Could you check a few things on this model? Use its own coordinates, in mm. A direction names the side the tool comes from. Give positions to 0.01 mm unless a question says otherwise; leave off trailing zeros. Order: outer loops, then holes, each group sorted by start corner. A loop starts at its lowest first (then second) coordinate and runs counter-clockwise, first axis right, second up. Notation, with made-up numbers: (69.25, 26) -> (95.25, 26) arc R22 ccw to (95.25, 64) -> close; hole circle Ø11 at (78, -27). An arc over 180 degrees is marked (long way). One line per item, written item: value.
```python
from build123d import *

# Parameters (mm, degrees)
SKETCH_1_R               = 18.75
EXTRUDE_1_DEPTH          = 60
SKETCH_2_R               = 6
EXTRUDE_2_DEPTH          = 5
SKETCH_3_R               = 3
EXTRUDE_3_DEPTH          = 15.5
SKETCH_4_W               = 7.331861777
SKETCH_4_H               = 1.908292791
CUT_EXTRUDE_1_DEPTH      = 14.5
PATTERN_CIRCULAR_1_COUNT = 6


with BuildPart() as part:
    # 草图1 → 凸台-拉伸1 (new body)
    with BuildSketch(Plane.XY):
        Circle(SKETCH_1_R)
    extrude(amount=EXTRUDE_1_DEPTH)

    # 草图2 → 凸台-拉伸2 (add)
    with BuildSketch(Plane.XY.offset(60)):
        with Locations((0, 7)):
            Circle(SKETCH_2_R)
    extrude(amount=EXTRUDE_2_DEPTH)

    # 草图3 → 凸台-拉伸3 (add)
    with BuildSketch(Plane.XY.offset(65)):
        with Locations((0, 7)):
            Circle(SKETCH_3_R)
    extrude(amount=EXTRUDE_3_DEPTH)

    # 草图4 → 切除-拉伸1 (cut)
    with BuildSketch(Plane.XY.offset(80.5)):
        with Locations((-0.04202298, 10.454146396)):
            Rectangle(SKETCH_4_W, SKETCH_4_H)
    extrude(amount=-CUT_EXTRUDE_1_DEPTH, mode=Mode.SUBTRACT)

    # 草图6 → M3 螺纹孔1 (revolve, cut)
    with BuildSketch(Plane(origin=(0, 15.5, 60), x_dir=(0, -1, 0), z_dir=(1, 0, 0))):
        Polygon((0, 0), (0, 8.251075774), (1.25, 7.5), (1.25, 0), align=None)
    hole_wizard_m3_1 = revolve(axis=Axis((0, 15.5, 66.35), (0, 0, -1)), mode=Mode.SUBTRACT)

    # 阵列(圆周)1: M3 螺纹孔1 ×6 about axis
    pattern_circular_1_axis = Axis((0, 0, 0), (0, 0, 1))
    for i in range(1, PATTERN_CIRCULAR_1_COUNT):
        add(hole_wizard_m3_1.rotate(pattern_circular_1_axis, i * 360 / PATTERN_CIRCULAR_1_COUNT), mode=Mode.SUBTRACT)


solid = part.part
```
1) For P1, Ø1.5, axis at x = 0, y = 15.5, coming from the +Z side; P2, Ø8, axis at x = -7, z = 45, coming from the +Y side; P3, Ø2.5, axis at x = 0, z = 71.5, coming from the +Y side, each with a flat end and sliding along its axis, tell me the tip position at first contact or that it passes through.
Answer below:
P1: stops at z = 52.2
P2: stops at y = 18.51
P3: stops at y = 9.5
2) Suppose I cut it at D-D, the plane y = 0. Write out the boundary of the cut face in (x, z), then the cut area to 3 significant figures.
Answer below:
outline: (-18.75, 0) -> (18.75, 0) -> (18.75, 60) -> (-18.75, 60) -> close
area: 2,250 mm2
3) For faces 1 (the flat face through (0, 9.5, 73)), 2 (the flat face through (0, 0, 0)), 3 (the cylindrical face through (12.184, -7.587, 56.302)), which set-ups out of +Z, -Z, +X, -X, +Y, -Y let a thin tool reach every point of the face, with its end or its side?
Answer below:
face 1: +Z, +X, -X, +Y
face 2: -Z, +X, -X, +Y, -Y
face 3: +Z
4) Suppose I cut it at C-C, the plane x = 5. Write out the boundary of the cut face in (y, z).
Answer below:
outline: (-18.07, 0) -> (18.07, 0) -> (18.07, 60) -> (10.32, 60) -> (10.32, 65) -> (3.68, 65) -> (3.68, 60) -> (-18.07, 60) -> close
5) If I drill on line 1 along Y through (x, z) = (-14, 57); line 2 along X through (y, z) = (7.75, 56.5); line 3 along X through (y, z) = (-7, 57), over which ranges is the centre line in solid material (lowest first)?
Answer below:
line 1: y = -12.47 to -8.86, -6.64 to 6.64, 8.86 to 12.47
line 2: x = -17.07 to -14.67, -12.17 to 12.17, 14.67 to 17.07
line 3: x = -17.39 to -14.42, -12.42 to 12.42, 14.42 to 17.39
6) Suppose I cut it at B-B, the plane z = 64. Write out the boundary of the cut face in (x, y), then the cut area to 3 significant figures.
Answer below:
outline: circle Ø12 at (0, 7)
area: 113 mm2
7) We'd pull the mould along X, two halves only. Please class faces 4 (the cylindrical face through (-14.27, -6.83, 56.3)), 5 (the flat face through (1, 10, 65)), 6 (the cylindrical face through (-0.78, 12.95, 62.46)): +X half, -X half, draft (parallel to the pull), parting line (faces both ways), or undercut.
Answer below:
face 4: undercut
face 5: draft
face 6: parting line
8) Suppose I cut it at A-A, the plane y = 12. Write out the boundary of the cut face in (x, z), then the cut area to 3 significant figures.
Answer below:
outline: (-14.41, 0) -> (14.41, 0) -> (14.41, 60) -> (3.32, 60) -> (3.32, 65) -> (-3.32, 65) -> (-3.32, 60) -> (-14.41, 60) -> close
area: 1,760 mm2
